Model file for the job. Use its own axes, mm. A direction names the side the tool comes from. Round coordinates to 2 decimals unless told otherwise and drop trailing zeros. Loops run counter-clockwise (first coordinate to the right, second up) from the corner with the lowest first, then second, coordinate; pieces in that order, holes last. Notation, with made-up numbers: (27, 76.25) -> (31, 76.25) arc R18 cw to (31, 107.25) -> close; hole circle Ø3 at (14, 39.25). An arc over 180 degrees is marked (long way). Use a Markdown table: item, result.
from build123d import *

# Parameters (mm, degrees)
BOSS_EXTRUDE1_DEPTH = 8
CHAMFER5_SIZE       = 5
FILLET1_R           = 2.5
SKETCH2_R           = 1.5
CUT_EXTRUDE1_DEPTH  = 47.658332589
SKETCH3_R           = 1.75
CUT_EXTRUDE2_DEPTH  = 44.200115741
SKETCH5_W           = 7
SKETCH5_H           = 8
CUT_EXTRUDE3_DEPTH  = 15
CUT_EXTRUDE5_DEPTH  = 15


with BuildPart() as part:
    # Sketch1 → Boss-Extrude1 (new, symmetric)
    with BuildSketch(Plane.XY):
        Polygon((-36, 0), (-21, 0), (-21, 20.5), (21, 20.5), (21, 0), (36, 0), (36, 2.5), (28, 2.5), (28, 25), (-28, 25), (-28, 2.5), (-36, 2.5), align=None)
    extrude(amount=BOSS_EXTRUDE1_DEPTH, both=True)

    # Chamfer5
    chamfer5_edges = [part.edges().sort_by_distance(p)[0] for p in [
        (-28, 25, 0),
        (28, 25, 0),
        (21, 0, 0),
        (-21, 0, 0),
    ]]
    chamfer(chamfer5_edges, length=CHAMFER5_SIZE)

    # Fillet1
    fillet1_edges = [part.edges().sort_by_distance(p)[0] for p in [
        (-28, 2.5, 0),
        (28, 2.5, 0),
    ]]
    fillet(fillet1_edges, radius=FILLET1_R)

    # Sketch2 → Cut-Extrude1 (cut, through all)
    with BuildSketch(Plane.XY.offset(8)):
        with Locations((-24.75, 14.475)):
            Circle(SKETCH2_R)
        with Locations((-24.75, 5.725)):
            Circle(SKETCH2_R)
        with Locations((24.75, 14.475)):
            Circle(SKETCH2_R)
        with Locations((24.75, 5.725)):
            Circle(SKETCH2_R)
    extrude(amount=-CUT_EXTRUDE1_DEPTH, mode=Mode.SUBTRACT)

    # Sketch3 → Cut-Extrude2 (cut, through all)
    with BuildSketch(Plane(origin=(0, 2.5, 0), x_dir=(1, 0, 0), z_dir=(0, 1, 0))):
        with Locations(Location((32.5, 4, 0), (0, 0, 270))):
            Circle(SKETCH3_R)
        with Locations(Location((32.5, -4, 0), (0, 0, 270))):
            Circle(SKETCH3_R)
        with Locations(Location((-32.5, 4, 0), (0, 0, 270))):
            Circle(SKETCH3_R)
        with Locations(Location((-32.5, -4, 0), (0, 0, 270))):
            Circle(SKETCH3_R)
    extrude(amount=-CUT_EXTRUDE2_DEPTH, mode=Mode.SUBTRACT)

    # Sketch5 → Cut-Extrude3 (cut)
    with BuildSketch(Plane(origin=(0, 25, 0), x_dir=(1, 0, 0), z_dir=(0, 1, 0))):
        with Locations((24.5, 0)):
            Rectangle(SKETCH5_W, SKETCH5_H)
        with Locations((-24.5, 0)):
            Rectangle(SKETCH5_W, SKETCH5_H)
    extrude(amount=-CUT_EXTRUDE3_DEPTH, mode=Mode.SUBTRACT)

    # Sketch7 → Cut-Extrude5 (cut)
    with BuildSketch(Plane(origin=(0, 25, 0), x_dir=(1, 0, 0), z_dir=(0, 1, 0))):
        with BuildLine():
            Line((21, 4), (21, -4))
            ThreePointArc((21, -4), (17, 0), (21, 4))
        make_face()
        with BuildLine():
            Line((-21, 4), (-21, -4))
            ThreePointArc((-21, -4), (-17, 0), (-21, 4))
        make_face()
    extrude(amount=-CUT_EXTRUDE5_DEPTH, mode=Mode.SUBTRACT)


solid = part.part
Q1. Band-saw the part on A-A, the plane x = 32.5. Give the cut face in (y, z), plus the area to 3 significant figures.
Results list:
| item | result |
|---|---|
| outline | (0, -8) -> (2.5, -8) -> (2.5, -5.75) -> (0, -5.75) -> close; (0, -2.25) -> (2.5, -2.25) -> (2.5, 2.25) -> (0, 2.25) -> close; (0, 5.75) -> (2.5, 5.75) -> (2.5, 8) -> (0, 8) -> close |
| area | 22.5 mm² |
Q2. Drill centre lines: L1, parallel to X at y = 10.5, z = -5; L2, parallel to Z at x = -25, y = 12.5; L3, parallel to X at y = 0.9, z = -4. Where is each one in solid material? Low to high. Write a range as from..to.
Results list:
| item | result |
|---|---|
| L1 | x = -28..-21, 21..28 |
| L2 | z = -8..-4, 4..8 |
| L3 | x = -36..-34.25, -30.75..-25.1, 25.1..30.75, 34.25..36 |
Q3. Tool access for faces 4 (the face through (-25, 10, 0)), 5 (the face through (-28, 9, 0)), 6 (the face through (33, 2.5, 0)), 7 (the face through (21, 9, 0)), 8 (the face through (24, 18, 4)): list every direction of +Z, -Z, +X, -X, +Y, -Y with a clear straight run to the whole face (end or side of a thin tool).
Results list:
| item | result |
|---|---|
| face 4 | +X, -X, +Y |
| face 5 | +Z, -Z, -X, +Y |
| face 6 | +Z, -Z, +X, +Y |
| face 7 | +Z, -Z, -Y |
| face 8 | +X, +Y |
Q4. Pull direction Y, two halves, no side cores. Call faces 1 (the face through (26, 22, 6)), 2 (the face through (-25, 18, -4)), 3 (the face through (-25.856, 15.489, 6.028)): released by +Y, released by -Y, zero draft, split by the parting line, or undercut.
Results list:
| item | result |
|---|---|
| face 1 | released by +Y |
| face 2 | zero draft |
| face 3 | undercut |
Q5. Band-saw the part on B-B, the plane z = 0. Give the cut face in (x, y) (3 decimals).
Results list:
| item | result |
|---|---|
| outline | (-36, 0) -> (-26, 0) -> (-21, 5) -> (-21, 10) -> (-28, 10) -> (-28, 5) arc R2.5 cw to (-30.5, 2.5) -> (-36, 2.5) -> close; (-17, 20.5) -> (17, 20.5) -> (17, 25) -> (-17, 25) -> close; (21, 5) -> (26, 0) -> (36, 0) -> (36, 2.5) -> (30.5, 2.5) arc R2.5 cw to (28, 5) -> (28, 10) -> (21, 10) -> close; hole circle Ø3 at (-24.75, 5.725); hole circle Ø3 at (24.75, 5.725) |
Q6. Flat gauge pins, fed straight in: pin 1 (1.5 mm diameter, centred on x = -16, z = 3, fed in from -Y); pin 2 (6 mm diameter, centred on x = 32, z = 0, fed in from +Y); pin 3 (1.6 mm diameter, centred on x = -32.5, z = 2.5, fed in from +Y). Where does each tip first touch, or does it go through?
Results list:
| item | result |
|---|---|
| pin 1 | stops at y = 20.5 |
| pin 2 | stops at y = 3 |
| pin 3 | stops at y = 2.5 |
Q7. Band-saw the part on D-D, the plane y = 3.25. Give the cut face in (x, z).
Results list:
| item | result |
|---|---|
| outline | (-28.71, -8) -> (-22.75, -8) -> (-22.75, 8) -> (-28.71, 8) -> close; (22.75, -8) -> (28.71, -8) -> (28.71, 8) -> (22.75, 8) -> close |
Q8. Band-saw the part on C-C, the plane x = 24.75. Give the cut face in (y, z) (3 decimals).
Results list:
| item | result |
|---|---|
| outline | (1.25, -8) -> (4.225, -8) -> (4.225, 8) -> (1.25, 8) -> close; (7.225, -8) -> (12.975, -8) -> (12.975, -4) -> (10, -4) -> (10, 4) -> (12.975, 4) -> (12.975, 8) -> (7.225, 8) -> close; (15.975, -8) -> (23.25, -8) -> (23.25, -4) -> (15.975, -4) -> close; (15.975, 4) -> (23.25, 4) -> (23.25, 8) -> (15.975, 8) -> close |
